Build history of the part. All positions in model axes, mm. A direction names the side the tool comes from. Round coordinates to 2 decimals unless told otherwise and drop trailing zeros. Loops run counter-clockwise (first coordinate to the right, second up) from the corner with the lowest first, then second, coordinate; pieces in that order, holes last. Notation, with made-up numbers: (41.25, 84) - (82.25, 84) arc R21 cw to (82.25, 117) - close; hole circle Ø11 at (-29, -27). An arc over 180 degrees is marked (long way). Use a Markdown table: item, result.
from build123d import *
from build123d.topology import SkipClean

# Parameters (mm, degrees)
SKETCH2_R           = 5
BOSS_EXTRUDE1_DEPTH = 200
SKETCH3_W           = 25
SKETCH3_H           = 25
BOSS_EXTRUDE2_DEPTH = 25
SKETCH4_R           = 10
BOSS_EXTRUDE3_DEPTH = 20


with BuildPart() as part:
    # Sketch2 → Boss-Extrude1 (new body)
    with BuildSketch(Plane(origin=(0, 0, 0), x_dir=(1, 0, 0), z_dir=(0, 1, 0))):
        with Locations(Location((0, 0, 0), (0, 0, 270))):
            Circle(SKETCH2_R)
    extrude(amount=BOSS_EXTRUDE1_DEPTH)

    # Sketch3 → Boss-Extrude2 (add)
    with BuildSketch(Plane.XZ):
        Rectangle(SKETCH3_W, SKETCH3_H)
    extrude(amount=BOSS_EXTRUDE2_DEPTH)

    # Sketch4 → Boss-Extrude3 (add)
    with BuildSketch(Plane.ZY.offset(12.5)):
        with Locations((0, -12.5)):
            Circle(SKETCH4_R)
    extrude(amount=BOSS_EXTRUDE3_DEPTH)

    # Sketch6 → Revolve2 (revolve)
    with SkipClean():  # the faces are left unmerged after this step: merging them gives an invalid solid
        with BuildSketch(Plane(origin=(0, 0, 0), x_dir=(0, 0, -1), z_dir=(1, 0, 0))):
            with BuildLine():
                Line((-5, 200), (5, 200))
                ThreePointArc((5, 200), (0, 205), (-5, 200))
            make_face()
        revolve(axis=Axis((0, 200, 5), (0, 0, -1)))


solid = part.part
Q1. Drop flat-ended pins along their axis: pin 1 (1 mm diameter, centred on x = -9, z = -3.5, fed in from +Y); pin 2 (4 mm diameter, centred on y = 169, z = 5, fed in from +X); pin 3 (12 mm diameter, centred on y = 126.5, z = 1.5, fed in from -X). Give the stop position or say it passes through.
Results found:
| item | result |
|---|---|
| pin 1 | stops at y = 0 |
| pin 2 | stops at x = 4 |
| pin 3 | stops at x = -5 |
Q2. Cut at A-A, the plane y = -12.5. List the corners of the cut face in (x, z).
Results found:
| item | result |
|---|---|
| outline | (-32.5, -10) - (-12.5, -10) - (-12.5, -12.5) - (12.5, -12.5) - (12.5, 12.5) - (-12.5, 12.5) - (-12.5, 10) - (-32.5, 10) - close |
Q3. Cut at B-B, the plane z = 0. List the corners of the cut face in (x, y).
Results found:
| item | result |
|---|---|
| outline | (-32.5, -22.5) - (-12.5, -22.5) - (-12.5, -25) - (12.5, -25) - (12.5, 0) - (5, 0) - (5, 200) arc R5 ccw to (-5, 200) - (-5, 0) - (-12.5, 0) - (-12.5, -2.5) - (-32.5, -2.5) - close |
Q4. Cut at D-D, the plane x = 9. List the corners of the cut face in (y, z), plus the area to 3 significant figures.
Results found:
| item | result |
|---|---|
| outline | (-25, -12.5) - (0, -12.5) - (0, 12.5) - (-25, 12.5) - close |
| area | 625 mm2 |
Q5. Probe line 1 (Y direction, x = -8, z = -0.75); line 2 (Y direction, x = -23, z = -0.25); line 3 (X direction, y = 3.5, z = 4.5). List the from-to ranges inside material, lowest first.
Results found:
| item | result |
|---|---|
| line 1 | y = -25 to 0 |
| line 2 | y = -22.5 to -2.5 |
| line 3 | x = -2.18 to 2.18 |
Q6. Cut at C-C, the plane x = -20.5. List the corners of the cut face in (y, z).
Results found:
| item | result |
|---|---|
| outline | circle Ø20 at (-12.5, 0) |
Q7. Which spindle directions (+Z, -Z, +X, -X, +Y, -Y) get a long thin tool onto all of the face, cutting with end or side? Do faces 1 (the face through (12.5, -12, 0)), 2 (the face through (-22.36, -18.58, -7.94)), 3 (the face through (-4.88, 98.6, -1.08)). Say none if no direction does.
Results found:
| item | result |
|---|---|
| face 1 | +Z, -Z, +X, +Y, -Y |
| face 2 | -X |
| face 3 | +Y |
